Can you work these out from the model? Positions are in its coordinate system, mm. Round coordinates to 2 decimals unless told otherwise and drop trailing zeros. Loops run counter-clockwise (first coordinate to the right, second up) from the corner with the lowest first, then second, coordinate; pieces in that order, holes last. Notation, with made-up numbers: (59.5, -26.75) -> (107.5, -26.75) arc R25 ccw to (107.5, -7.75) -> close; hole circle Ø8 at (-10, 88.25). An arc over 180 degrees is marked (long way). Write item = value, one per line.
from build123d import *

# Parameters (mm, degrees)
PAD_DEPTH    = 2
SKETCH001_W  = 41.942294
SKETCH001_H  = 0.2
POCKET_DEPTH = 0.5


with BuildPart() as part:
    # Sketch → Pad (new body)
    with BuildSketch(Plane.XZ):
        Polygon((-20, 6.85827), (20, 6.85827), (0, 15.85827), align=None)
    extrude(amount=PAD_DEPTH)

    # Sketch001 (on Face5 of Pad) → Pocket (cut)
    with BuildSketch(Plane.XZ.offset(2)):
        with Locations((0.24899, 7.390751)):
            Rectangle(SKETCH001_W, SKETCH001_H)
        with Locations((0.253757, 8.087106)):
            Rectangle(SKETCH001_W, SKETCH001_H)
        with Locations((0.258524, 8.783461)):
            Rectangle(SKETCH001_W, SKETCH001_H)
        with Locations((0.263291, 9.479816)):
            Rectangle(SKETCH001_W, SKETCH001_H)
        with Locations((0.268058, 10.176171)):
            Rectangle(SKETCH001_W, SKETCH001_H)
        with Locations((0.272825, 10.872526)):
            Rectangle(SKETCH001_W, SKETCH001_H)
        with Locations((0.277592, 11.568881)):
            Rectangle(SKETCH001_W, SKETCH001_H)
        with Locations((0.282359, 12.265236)):
            Rectangle(SKETCH001_W, SKETCH001_H)
        with Locations((0.287126, 12.961591)):
            Rectangle(SKETCH001_W, SKETCH001_H)
        with Locations((0.291893, 13.657946)):
            Rectangle(SKETCH001_W, SKETCH001_H)
        with Locations((0.29666, 14.354301)):
            Rectangle(SKETCH001_W, SKETCH001_H)
        with Locations((0.301427, 15.050656)):
            Rectangle(SKETCH001_W, SKETCH001_H)
        with Locations((0.306194, 15.747011)):
            Rectangle(SKETCH001_W, SKETCH001_H)
    extrude(amount=-POCKET_DEPTH, mode=Mode.SUBTRACT)


solid = part.part
1. I'm going to push flat-ended pins straight in: pin 1 (0.6 mm diameter, centred on x = 1, y = -2, fed in from +Z); pin 2 (4 mm diameter, centred on x = -4, z = 14, fed in from +Y); pin 3 (0.6 mm diameter, centred on x = -1.5, y = -2, fed in from +Z). Where does each tip first touch, or does it pass through?
Entries:
pin_1 = 15.54
pin_2 = 0
pin_3 = 15.32
2. Suppose I cut it at A-A, the plane x = -15. List the corners of the cut face in (y, z) for me, and give its area (3 significant figures).
Entries:
outline = (-2, 6.86) -> (0, 6.86) -> (0, 9.11) -> (-2, 9.11) -> (-2, 8.88) -> (-1.5, 8.88) -> (-1.5, 8.68) -> (-2, 8.68) -> (-2, 8.19) -> (-1.5, 8.19) -> (-1.5, 7.99) -> (-2, 7.99) -> (-2, 7.49) -> (-1.5, 7.49) -> (-1.5, 7.29) -> (-2, 7.29) -> close
area = 4.20 mm²
3. Suppose I cut it at B-B, the plane y = -1.05. List the corners of the cut face in (x, z) for me.
Entries:
outline = (-20, 6.86) -> (20, 6.86) -> (0, 15.86) -> close
4. I need wall thicknesses on line 1 (Y direction, x = 3, z = 11.5); line 2 (X direction, y = -1.7, z = 8.25); line 3 (Z direction, x = 6.5, y = -0.85). Which ranges of each line are inside material? Lowest first, please. Write a range as [from, to].
Entries:
line_1 = [-1.5, 0]
line_2 = [-16.91, 16.91]
line_3 = [6.86, 12.93]
